Input: part model. Units: mm. Frame: model coordinates. Coordinates: 2 decimals unless noted, no trailing zeros. Order: outer loops, then holes, each group sorted by start corner. A loop starts at its lowest first (then second) coordinate and runs counter-clockwise, first axis right, second up. Notation, with made-up numbers: M 1,59 L 21,59 A20 ccw 21,76 Z; hole C 28.5,-3.5 d4. An arc over 180 degrees is marked long. Answer in a Markdown table with one row per item.
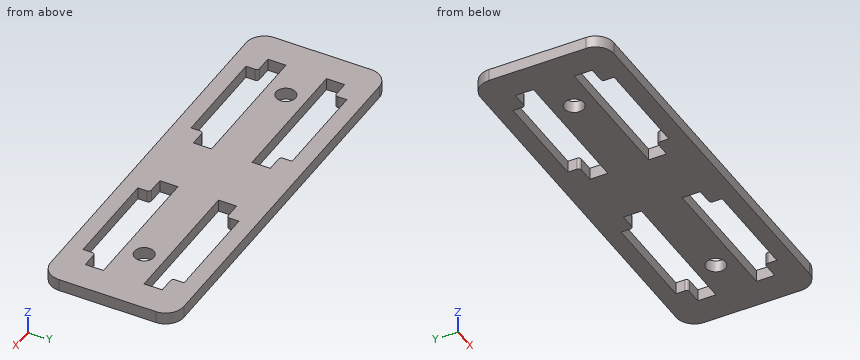
from build123d import *

# Parameters (mm, degrees)
SKETCH_1_R      = 1.6
EXTRUDE_1_DEPTH = 2


with BuildPart() as part:
    # 草图1 → 凸台-拉伸1 (new body)
    with BuildSketch(Plane.XY):
        with BuildLine():
            Line((-29.812520549, 11), (29.812520549, 11))
            ThreePointArc((29.812520549, 11), (31.933840892, 10.121320344), (32.812520549, 8))
            Line((32.812520549, 8), (32.812520549, -8))
            ThreePointArc((32.812520549, -8), (31.933840892, -10.121320344), (29.812520549, -11))
            Line((29.812520549, -11), (-29.812520549, -11))
            ThreePointArc((-29.812520549, -11), (-31.933840892, -10.121320344), (-32.812520549, -8))
            Line((-32.812520549, -8), (-32.812520549, 8))
            ThreePointArc((-32.812520549, 8), (-31.933840892, 10.121320344), (-29.812520549, 11))
        make_face()
        with Locations((-21.602967139, 3e-09)):
            Circle(SKETCH_1_R, mode=Mode.SUBTRACT)
        with Locations(Location((21.602967139, 3e-09, 0), (0, 0, 180))):
            Circle(SKETCH_1_R, mode=Mode.SUBTRACT)
        with BuildLine():
            Line((-27.82296712, -6.350000006), (-25.322967139, -6.350000006))
            ThreePointArc((-25.322967139, -6.350000006), (-24.969413752, -6.496446613), (-24.822967144, -6.850000001))
            Line((-24.822967144, -6.850000001), (-24.822967144, -8.350000009))
            Line((-24.822967144, -8.350000009), (-8.122967147, -8.350000009))
            Line((-8.122967147, -8.350000009), (-8.122967147, -6.850000006))
            ThreePointArc((-8.122967147, -6.850000006), (-7.976520539, -6.496446619), (-7.622967152, -6.350000011))
            Line((-7.622967152, -6.350000011), (-5.122967162, -6.350000011))
            Line((-5.122967162, -6.350000011), (-5.122967162, -3.349999976))
            Line((-5.122967162, -3.349999976), (-27.82296712, -3.349999976))
            Line((-27.82296712, -3.349999976), (-27.82296712, -6.350000006))
        make_face(mode=Mode.SUBTRACT)
        with BuildLine():
            Line((-8.12296715, 8.350000017), (-24.822967148, 8.350000017))
            Line((-24.822967148, 8.350000017), (-24.822967148, 6.850000008))
            ThreePointArc((-24.822967148, 6.850000008), (-24.969413756, 6.496446621), (-25.322967143, 6.350000013))
            Line((-25.322967143, 6.350000013), (-27.822967124, 6.350000013))
            Line((-27.822967124, 6.350000013), (-27.822967124, 3.349999975))
            Line((-27.822967124, 3.349999975), (-5.122967149, 3.349999975))
            Line((-5.122967149, 3.349999975), (-5.122967149, 6.350000013))
            Line((-5.122967149, 6.350000013), (-7.622967155, 6.350000013))
            ThreePointArc((-7.622967155, 6.350000013), (-7.976520542, 6.496446621), (-8.12296715, 6.850000008))
            Line((-8.12296715, 6.850000008), (-8.12296715, 8.350000017))
        make_face(mode=Mode.SUBTRACT)
        with BuildLine():
            Line((24.822967148, 8.350000017), (24.822967148, 6.850000008))
            ThreePointArc((24.822967148, 6.850000008), (24.969413756, 6.496446621), (25.322967143, 6.350000013))
            Line((25.322967143, 6.350000013), (27.822967124, 6.350000013))
            Line((27.822967124, 6.350000013), (27.822967124, 3.349999975))
            Line((27.822967124, 3.349999975), (5.122967149, 3.349999975))
            Line((5.122967149, 3.349999975), (5.122967149, 6.350000013))
            Line((5.122967149, 6.350000013), (7.622967155, 6.350000013))
            ThreePointArc((7.622967155, 6.350000013), (7.976520542, 6.496446621), (8.12296715, 6.850000008))
            Line((8.12296715, 6.850000008), (8.12296715, 8.350000017))
            Line((8.12296715, 8.350000017), (24.822967148, 8.350000017))
        make_face(mode=Mode.SUBTRACT)
        with BuildLine():
            Line((24.822967144, -6.850000001), (24.822967144, -8.350000009))
            Line((24.822967144, -8.350000009), (8.122967147, -8.350000009))
            Line((8.122967147, -8.350000009), (8.122967147, -6.850000006))
            ThreePointArc((8.122967147, -6.850000006), (7.976520539, -6.496446619), (7.622967152, -6.350000011))
            Line((7.622967152, -6.350000011), (5.122967162, -6.350000011))
            Line((5.122967162, -6.350000011), (5.122967162, -3.349999976))
            Line((5.122967162, -3.349999976), (27.82296712, -3.349999976))
            Line((27.82296712, -3.349999976), (27.82296712, -6.350000006))
            Line((27.82296712, -6.350000006), (25.322967139, -6.350000006))
            ThreePointArc((25.322967139, -6.350000006), (24.969413752, -6.496446613), (24.822967144, -6.850000001))
        make_face(mode=Mode.SUBTRACT)
    extrude(amount=EXTRUDE_1_DEPTH)


solid = part.part
1) Cut plane B-B, the plane y = 0. Output: boundary loops of the cut face in (x, z), and give its area (3 significant figures).
Resolved:
| item | result |
|---|---|
| outline | M -32.81,0 L -23.2,0 L -23.2,2 L -32.81,2 Z; M -20,0 L 20,0 L 20,2 L -20,2 Z; M 23.2,0 L 32.81,0 L 32.81,2 L 23.2,2 Z |
| area | 118 mm2 |
2) Cut plane A-A, the plane x = 15. Output: boundary loops of the cut face in (y, z).
Resolved:
| item | result |
|---|---|
| outline | M -11,0 L -8.35,0 L -8.35,2 L -11,2 Z; M -3.35,0 L 3.35,0 L 3.35,2 L -3.35,2 Z; M 8.35,0 L 11,0 L 11,2 L 8.35,2 Z |
3) Material intervals for probe 1 along Y at (x, z) = (-26, 1.35); probe 2 along X at (y, z) = (-5.75, 1.9); probe 3 along X at (y, z) = (-6.75, 1.3), sorted ascending.
Resolved:
| item | result |
|---|---|
| probe 1 | y = -11 to -6.35, -3.35 to 3.35, 6.35 to 11 |
| probe 2 | x = -32.81 to -27.82, -5.12 to 5.12, 27.82 to 32.81 |
| probe 3 | x = -32.81 to -24.83, -8.11 to 8.11, 24.83 to 32.81 |
4) Cut plane C-C, the plane z = 1.65. State how many separate pieces and enclosed holes the cut face has, and give its area (3 significant figures).
Resolved:
| item | result |
|---|---|
| separate pieces | 1 |
| enclosed holes | 6 |
| area | 1,010 mm2 |
